Design review of the part shown in the three views and the two pictorial views. Dimensions are in mm from the part's minimum x, y and z. A direction names the side the tool comes from. Coordinates: 2 decimals unless noted, no trailing zeros. Loops run counter-clockwise (first coordinate to the right, second up) from the corner with the lowest first, then second, coordinate; pieces in that order, holes last. Notation, with made-up numbers: M 68,47.5 L 94,47.5 A28 ccw 94,73.5 Z; hole C 74.5,16 d2. An arc over 180 degrees is marked long. Use one line per item in the form item = value.
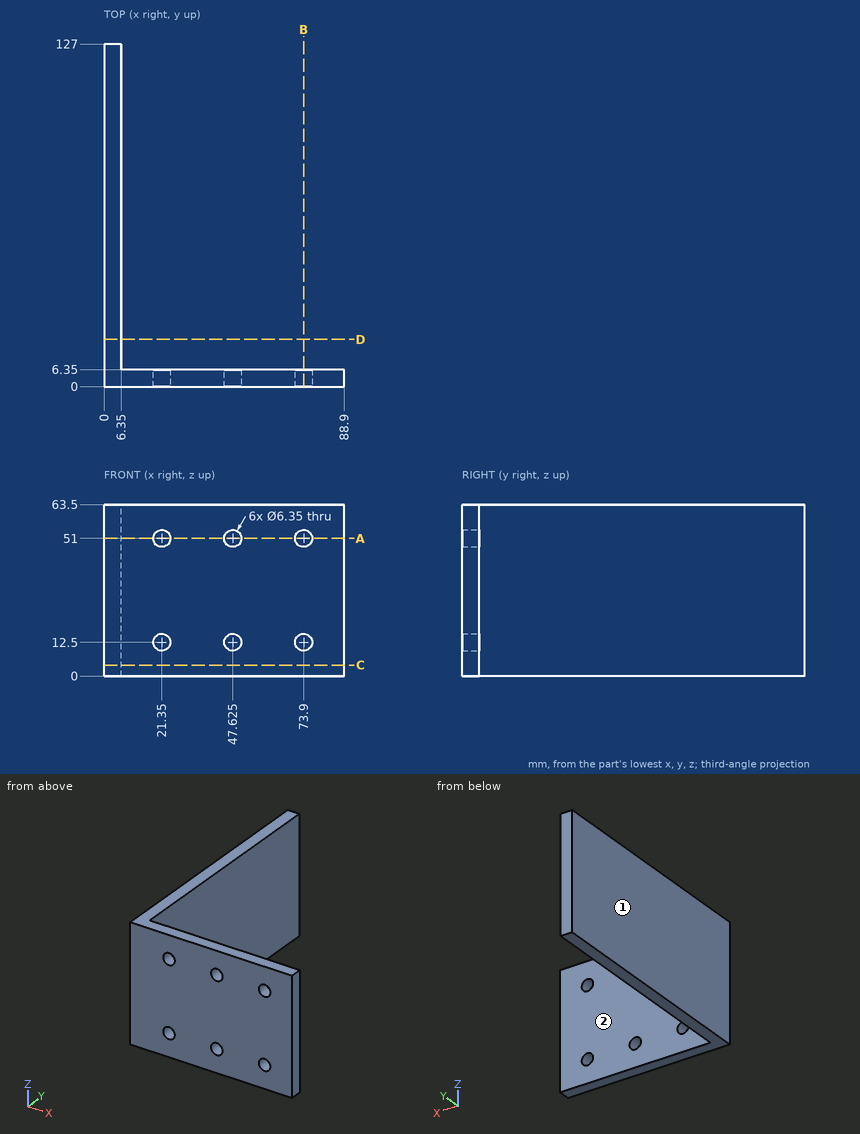
1. Machinability: for the marked faces 1 and 2, which of the approach directions +Z, -Z, +X, -X, +Y, -Y give a long, thin tool a straight path to every point of the face, cutting with its end or side? Answer none if there is none.
Response values:
face_1 = +Z, -Z, -X, +Y, -Y
face_2 = +Z, -Z, +X, +Y
2. Add section A-A (z = 51). State the section outline as (x, y) points (3 decimals), then the cut area to 3 significant figures.
Response values:
outline = M 0,0 L 18.175,0 L 18.175,6.35 L 6.35,6.35 L 6.35,127 L 0,127 Z; M 24.525,0 L 44.45,0 L 44.45,6.35 L 24.525,6.35 Z; M 50.8,0 L 70.725,0 L 70.725,6.35 L 50.8,6.35 Z; M 77.075,0 L 88.9,0 L 88.9,6.35 L 77.075,6.35 Z
area = 1,210 mm^2
3. Add section C-C (z = 4). State the section outline as (x, y) points, then the cut area to 3 significant figures.
Response values:
outline = M 0,0 L 88.9,0 L 88.9,6.35 L 6.35,6.35 L 6.35,127 L 0,127 Z
area = 1,330 mm^2
4. Add section B-B (x = 73.9). State the section outline as (y, z) points (3 decimals), then the cut area to 3 significant figures.
Response values:
outline = M 0,0 L 6.35,0 L 6.35,9.325 L 0,9.325 Z; M 0,15.675 L 6.35,15.675 L 6.35,47.825 L 0,47.825 Z; M 0,54.175 L 6.35,54.175 L 6.35,63.5 L 0,63.5 Z
area = 323 mm^2
5. Add section D-D (y = 17.5). State the section outline as (x, z) points, then the cut area to 3 significant figures.
Response values:
outline = M 0,0 L 6.35,0 L 6.35,63.5 L 0,63.5 Z
area = 403 mm^2
6. Wall thickness on line 1 along Z through (x, y) = (21.35, 3) (3 decimals); line 2 along X through (y, z) = (4.25, 51) (3 decimals); line 3 along Z through (x, y) = (73, 4): over which ranges is each line inside the solid? List them lowest first. Write a range as from..to.
Response values:
line_1 = 0..9.325, 15.675..47.825, 54.175..63.5
line_2 = 0..18.175, 24.525..44.45, 50.8..70.725, 77.075..88.9
line_3 = 0..9.46, 15.54..47.96, 54.04..63.5
7. Insertion check: P1, Ø4, axis at y = 67.5, z = 8, coming from the +X side; P2, Ø3, axis at x = 41.5, z = 38, coming from the +Y side. Each pin has a flat end and moves straight along its axis. Give the tip position at first contact, or say it passes through.
Response values:
P1 = 6.35
P2 = 6.35
